from build123d import *

# Parameters (mm, degrees)
BASE_FLANGE1_DEPTH = 2.65684
FILLET1_R          = 3.175


# Sheet-metal steps are written as plain solids
with BuildPart() as part:
    # Sketch1 → Base-Flange1 (new body)
    with BuildSketch(Plane.XY):
        with BuildLine():
            Line((-180.45684, 0), (-15.24, 0))
            ThreePointArc((-15.24, 0), (0, 15.24), (15.24, 0))
            Line((15.24, 0), (180.45684, 0))
            ThreePointArc((180.45684, 0), (143.97849234, 108.788165011), (49.29124, 173.594483674))
            Line((49.29124, 173.594483674), (49.29124, 249.794483674))
            Line((49.29124, 249.794483674), (114.598461144, 327.624599095))
            Line((114.598461144, 327.624599095), (-114.598461144, 327.624599095))
            Line((-114.598461144, 327.624599095), (-49.29124, 249.794483674))
            Line((-49.29124, 249.794483674), (-49.29124, 173.594483674))
            ThreePointArc((-49.29124, 173.594483674), (-143.97849234, 108.788165011), (-180.45684, 0))
        make_face()
    extrude(amount=-BASE_FLANGE1_DEPTH)

    # Fillet1
    fillet1_edges = [part.edges().sort_by_distance(p)[0] for p in [
        (-49.29124, 173.594483674, -1.32842),
        (-49.29124, 249.794483674, -1.32842),
        (49.29124, 249.794483674, -1.32842),
        (49.29124, 173.594483674, -1.32842),
    ]]
    fillet(fillet1_edges, radius=FILLET1_R)


solid = part.part
Here's how the part is built. I have some questions about the finished solid (model axes, mm). A direction names the side the tool comes from. Give positions to 0.01 mm unless a question says otherwise; leave off trailing zeros. Order: outer loops, then holes, each group sorted by start corner. A loop starts at its lowest first (then second) coordinate and runs counter-clockwise, first axis right, second up. Notation, with made-up numbers: M 85.5,59 L 96.5,59 A25 ccw 96.5,81 Z; hole C -10.5,-27.75 d2. An arc over 180 degrees is marked long. Answer as a JSON object with one key per item and string values. Group by question number.
1) I'm going to push flat-ended pins straight in: pin 1 Ø1.3 at (y, z) = (227, -1.5) entering from -X; pin 2 Ø1.3 at (y, z) = (222.5, -1) entering from +X. Where does each tip first touch, or does it pass through?
2) Suppose I cut it at A-A, the plane z = -0.75. Write out the boundary of the cut face in (x, y) (3 decimals).
3) On a 3-axis mill with a long thin cutter (end or side, diameter ignored), from which of +Z, -Z, +X, -X, +Y, -Y can I reach the whole of each face in a straight line? I mean faces 1 (the flat face through (81.86, 288.61, -1.31)), 2 (the flat face through (-3, 130, -2.657)), 3 (the cylindrical face through (-143.71, 109.14, -1.31)). Say none if no direction works.
4) Please list where these lines run through material, in increasing order: L1, parallel to X at y = 181, z = -2.4; L2, parallel to Y at x = 109, z = -2.25; L3, parallel to Y at x = 79, z = -0.9. Write a range as [from, to].
5) Suppose I cut it at C-C, the plane y = 190. Write out the boundary of the cut face in (x, z).
6) Suppose I cut it at B-B, the plane x = 0. Write out the boundary of the cut face in (y, z), plus the area to 3 significant figures.
7) We'd pull the mould along X, two halves only. Please class faces 4 (the cylindrical face through (-0.335, 15.236, -1.31)), 5 (the flat face through (-3, 130, 0)), 6 (the cylindrical face through (145.65, 106.54, -1.31)): pulls with the +X half, pulls with the -X half, needs draft (parallel to the pull), parting line crosses it, or undercut.
Results found:
{
 "1": {"pin 1": "x = -49.29", "pin 2": "x = 49.29"},
 "2": {"outline": "M -180.457,0 L -15.24,0 A15.24 cw 15.24,0 L 180.457,0 A180.457 ccw 51.559,172.934 A3.175 cw 49.291,175.977 L 49.291,248.639 A3.175 cw 50.034,250.68 L 114.598,327.625 L -114.598,327.625 L -50.034,250.68 A3.175 cw -49.291,248.639 L -49.291,175.977 A3.175 cw -51.559,172.934 A180.457 ccw Z"},
 "3": {"face 1": "+Z, -Z, +X", "face 2": "-Z, +X, -X, +Y, -Y", "face 3": "+Z, -Z, -X"},
 "4": {"L1": "[-49.29, 49.29]", "L2": "[0, 143.82], [320.95, 327.62]", "L3": "[0, 162.25], [285.2, 327.62]"},
 "5": {"outline": "M -49.29,-2.66 L 49.29,-2.66 L 49.29,0 L -49.29,0 Z"},
 "6": {"outline": "M 15.24,-2.66 L 327.62,-2.66 L 327.62,0 L 15.24,0 Z", "area": "830 mm²"},
 "7": {"face 4": "undercut", "face 5": "needs draft", "face 6": "pulls with the +X half"}
}
